Part model, mm, in its own coordinate system. Round coordinates to 2 decimals unless told otherwise and drop trailing zeros. Loops run counter-clockwise (first coordinate to the right, second up) from the corner with the lowest first, then second, coordinate; pieces in that order, holes last.
from build123d import *

# Parameters (mm, degrees)
SKETCH_R  = 2.1
PAD_DEPTH = 1


with BuildPart() as part:
    # Sketch → Pad (new body)
    with BuildSketch(Plane.XY):
        with BuildLine():
            ThreePointArc((0, 5), (-5, 0), (0, -5))
            Line((0, -5), (20, -5))
            ThreePointArc((20, -5), (25, 0), (20, 5))
            Line((0, 5), (20, 5))
        make_face()
        Circle(SKETCH_R, mode=Mode.SUBTRACT)
        with Locations((10, 0)):
            Circle(SKETCH_R, mode=Mode.SUBTRACT)
        with Locations((20, 0)):
            Circle(SKETCH_R, mode=Mode.SUBTRACT)
    extrude(amount=PAD_DEPTH)


solid = part.part
1) Slice it at A-A, the plane x = 10. Give the cut face in (y, z).
Values:
outline: (-5, 0) - (-2.1, 0) - (-2.1, 1) - (-5, 1) - close; (2.1, 0) - (5, 0) - (5, 1) - (2.1, 1) - close
2) Mould opens along X. For faces 1 (the face through (9.8, 2.3, 1)), 2 (the face through (2.003, 0.631, 0.493)), 3 (the face through (25, -0.1, 0.5)) say: released by +X, released by -X, zero draft, split by the parting line, or undercut.
Values:
face 1: zero draft
face 2: undercut
face 3: released by +X
3) Drop a flat-ended pin along its axis: pin 1 Ø3.5 at (x, y) = (0, 0) entering from -Z. Give the stop position or say it passes through.
Values:
pin 1: passes through
4) Slice it at D-D, the plane x = -0.5. Give the cut face in (y, z), then the cut area to 3 significant figures.
Values:
outline: (-4.97, 0) - (-2.04, 0) - (-2.04, 1) - (-4.97, 1) - close; (2.04, 0) - (4.97, 0) - (4.97, 1) - (2.04, 1) - close
area: 5.87 mm2
5) Wall check: line 1 along Y through (x, z) = (20, 0.55); line 2 along X through (y, z) = (-1, 0.9); line 3 along X through (y, z) = (1.5, 0.5). Give the ranges that are in metal, low to high.
Values:
line 1: y = -5 to -2.1, 2.1 to 5
line 2: x = -4.9 to -1.85, 1.85 to 8.15, 11.85 to 18.15, 21.85 to 24.9
line 3: x = -4.77 to -1.47, 1.47 to 8.53, 11.47 to 18.53, 21.47 to 24.77
6) Slice it at C-C, the plane z = 0.75. Give the cut face in (x, y).
Values:
outline: (0, -5) - (20, -5) arc R5 ccw to (20, 5) - (0, 5) arc R5 ccw to start; hole circle Ø4.2 at (0, 0); hole circle Ø4.2 at (10, 0); hole circle Ø4.2 at (20, 0)
7) Slice it at B-B, the plane y = 1.5. Give the cut face in (x, z), then the cut area to 3 significant figures.
Values:
outline: (-4.77, 0) - (-1.47, 0) - (-1.47, 1) - (-4.77, 1) - close; (1.47, 0) - (8.53, 0) - (8.53, 1) - (1.47, 1) - close; (11.47, 0) - (18.53, 0) - (18.53, 1) - (11.47, 1) - close; (21.47, 0) - (24.77, 0) - (24.77, 1) - (21.47, 1) - close
area: 20.7 mm2
